from build123d import *

# Parameters (mm, degrees)
ESQUISSE1_R             = 5
BOSS_EXTRU_1_DEPTH      = 1
ESQUISSE2_R             = 4
BOSS_EXTRU_2_DEPTH      = 8
ESQUISSE3_R             = 1.65
ENL_V_MAT_EXTRU_1_DEPTH = 7


with BuildPart() as part:
    # Esquisse1 → Boss.-Extru.1 (new body)
    with BuildSketch(Plane.XY):
        Circle(ESQUISSE1_R)
    extrude(amount=BOSS_EXTRU_1_DEPTH)

    # Esquisse2 → Boss.-Extru.2 (add)
    with BuildSketch(Plane.XY.offset(1)):
        Circle(ESQUISSE2_R)
    extrude(amount=BOSS_EXTRU_2_DEPTH)

    # Esquisse3 → Enlèv. mat.-Extru.1 (cut)
    with BuildSketch(Plane.XY.offset(9)):
        with Locations((1.5, 0)):
            Circle(ESQUISSE3_R)
    extrude(amount=-ENL_V_MAT_EXTRU_1_DEPTH, mode=Mode.SUBTRACT)


solid = part.part
The model under review builds one solid part; all positions refer to its coordinate system, in mm. Round coordinates to 2 decimals unless told otherwise and drop trailing zeros. Order: outer loops, then holes, each group sorted by start corner. A loop starts at its lowest first (then second) coordinate and runs counter-clockwise, first axis right, second up. Notation, with made-up numbers: (22, 51.25) - (81, 51.25) arc R14 cw to (81, 64.25) - close; hole circle Ø5 at (-34, 80.5). An arc over 180 degrees is marked (long way). Use one line per item in the form item = value.
Q1. Add section C-C on z = 0.5. Give the boundary of the cut face in (x, y).
Response values:
outline = circle Ø10 at (0, 0)
Q2. Clearance check with flat-ended pins moving along their axes: P1, Ø4, axis at y = 1, z = 8, coming from the -X side; P2, Ø1, axis at x = 1.5, y = 0, coming from the +Z side; P3, Ø3, axis at x = 2.5, z = 4.5, coming from the +Y side. State where each tip first meets the part, or that it passes through.
Response values:
P1 = -4
P2 = 2
P3 = 3.87
Q3. Mouldability with a two-part tool opening along X and no side actions: class faces 1 (the cylindrical face through (-0.867, -3.905, 4.944)), 2 (the flat face through (1, 0, 2)), 3 (the flat face through (0, 0, 0)), 4 (the cylindrical face through (3.074, 0.496, 5.549)) as pulls with the +X half, pulls with the -X half, needs draft (parallel to the pull), parting line crosses it, or undercut.
Response values:
face_1 = parting line crosses it
face_2 = undercut
face_3 = needs draft
face_4 = undercut
Q4. To check wall thickness, follow line 1 (Z direction, x = -3, y = -2.75); line 2 (Y direction, x = 1.5, z = 7.25); line 3 (Z direction, x = 0, y = 0). State the ranges of each line that lie inside material, in increasing order.
Response values:
line_1 = 0 to 1
line_2 = -3.71 to -1.65, 1.65 to 3.71
line_3 = 0 to 2
Q5. Add section A-A on y = 0. Give the boundary of the cut face in (x, z).
Response values:
outline = (-5, 0) - (5, 0) - (5, 1) - (4, 1) - (4, 9) - (3.15, 9) - (3.15, 2) - (-0.15, 2) - (-0.15, 9) - (-4, 9) - (-4, 1) - (-5, 1) - close
Q6. Add section D-D on z = 2.75. Give the boundary of the cut face in (x, y).
Response values:
outline = circle Ø8 at (0, 0); hole circle Ø3.3 at (1.5, 0)
Q7. Add section B-B on x = 2. Give the boundary of the cut face in (y, z), then the cut area to 3 significant figures.
Response values:
outline = (-4.58, 0) - (4.58, 0) - (4.58, 1) - (3.46, 1) - (3.46, 9) - (1.57, 9) - (1.57, 2) - (-1.57, 2) - (-1.57, 9) - (-3.46, 9) - (-3.46, 1) - (-4.58, 1) - close
area = 42.6 mm^2
